Input: part model. Units: mm. Frame: model coordinates. Round coordinates to 2 decimals unless told otherwise and drop trailing zeros. Loops run counter-clockwise (first coordinate to the right, second up) from the corner with the lowest first, then second, coordinate; pieces in that order, holes last. Notation, with made-up numbers: (21, 7.5) - (35, 7.5) arc R22 ccw to (35, 14.5) - close; hole circle Ø8 at (9.5, 21). An arc over 180 degrees is marked (long way). Use CSV: the item, a comma, the result in double quotes. Start each with the question number.
1. Cut plane B-B (z = -9). Return loops of the section in (x, y), and give its area (3 significant figures).
2. Cut plane A-A (y = 8). Return loops of the section in (x, z).
3. Pin query (flat end, axial travel): P1, Ø1.5, axis at x = 7, z = -5, coming from the +Y side; P2, Ø6, axis at y = 6, z = 2, coming from the -X side; P3, Ø5, axis at x = 6.5, y = 7.5, coming from the -Z side. Return the tip coordinate at first contact, or that it passes through.
4. Material intervals for probe 1 along Y at (x, z) = (5.5, 0.5) (3 decimals); probe 2 along Y at (x, z) = (-0.25, 7.75); probe 3 along Z at (x, y) = (-7.25, 5.5), sorted ascending. Write a range as from..to.
```python
from build123d import *

# Parameters (mm, degrees)
ENL_V_MAT_EXTRU_2_DEPTH = 11.698916896
ENL_V_MAT_EXTRU_4_DEPTH = 3
ENL_V_MAT_EXTRU_4_TAPER = 5


with BuildPart() as part:
    # Esquisse1 → Révol.-Mince1 (revolve)
    with BuildSketch(Plane.XY):
        with BuildLine():
            ThreePointArc((0, 10.698916896), (10.698916896, 0), (0, -10.698916896))
            Line((0, -10.698916896), (0, -0.698916896))
            ThreePointArc((0, -0.698916896), (0.698916896, 0), (0, 0.698916896))
            Line((0, 0.698916896), (0, 10.698916896))
        make_face()
    revolve(axis=Axis((0, -3.545926921, 0), (0, 1, 0)))

    # Esquisse2 → Enlèv. mat.-Extru.2 (cut, through all)
    with BuildSketch(Plane.XY):
        with BuildLine():
            Line((-9.498856237, -1.25), (-9.5, -1))
            add(Edge.make_bspline(
                [(-9.5, -1), (0, 1), (9.5, -1)],
                knots=[0, 0, 0, 1, 1, 1], degree=2))
            Line((9.5, -1), (9.501143763, -1.25))
            add(Edge.make_bspline(
                [(-9.498856237, -1.25), (0.001143763, 0.750101861), (9.501143763, -1.25)],
                knots=[0, 0, 0, 1, 1, 1], degree=2))
        make_face()
    extrude(amount=ENL_V_MAT_EXTRU_2_DEPTH, mode=Mode.SUBTRACT)

    # Esquisse4 → Enlèv. mat.-Extru.4 (cut)
    with BuildSketch(Plane.XY.offset(10)):
        Polygon((3.719730148, -0.25), (6.452328662, -2.65272264), (8.21328513, -0.65), align=None)
        Polygon((-6.452328662, -2.65272264), (-3.719730148, -0.25), (-8.21328513, -0.65), align=None)
    extrude(amount=-ENL_V_MAT_EXTRU_4_DEPTH, taper=ENL_V_MAT_EXTRU_4_TAPER, mode=Mode.SUBTRACT)


solid = part.part
```
Established:
1,outline,"circle Ø11.57 at (0, 0)"
1,area,"105 mm2"
2,outline,"circle Ø14.21 at (0, 0)"
3,P1,"stops at y = 7.27"
3,P2,"stops at x = -10.17"
3,P3,"stops at z = -7.7"
4,probe 1,"y = -9.163..-0.585, -0.335..9.163"
4,probe 2,"y = -7.37..-0.25, 0..7.37"
4,probe 3,"z = -5.63..5.63"
